from build123d import *

# Parameters (mm, degrees)
F0_R     = 31.75
F0_R_2   = 3.81
F1_DEPTH = 12.7
F4_DEPTH = 12.7
F5_COUNT = 20


with BuildPart() as f1:
    # F0 (on Front) → F1 (new body)
    with BuildSketch(Plane.XZ):
        Circle(F0_R)
        Circle(F0_R_2, mode=Mode.SUBTRACT)
    extrude(amount=F1_DEPTH)

    # F2 (on face) → F4 (join, through all)
    with BuildSketch(Plane.XZ.offset(12.7)):
        with BuildLine():
            Line((1.376606524, 33.9144617319), (0, 31.75))
            ThreePointArc((0, 31.75), (1.1215923583, 31.7301832737), (2.2417846354, 31.6707578319))
            Line((2.2417846354, 31.6707578319), (1.376606524, 33.9144617319))
        make_face()
    extrude(amount=-F4_DEPTH)

    # F5: F1 ×20 about axis
    f5_axis = Axis((0, -7.9411361367, 0), (0, -1, 0))


with BuildPart() as f1_1:
    add(f1.part)
    for i in range(1, F5_COUNT):
        add(f1.part.rotate(f5_axis, i * 360 / F5_COUNT))


solid = f1_1.part
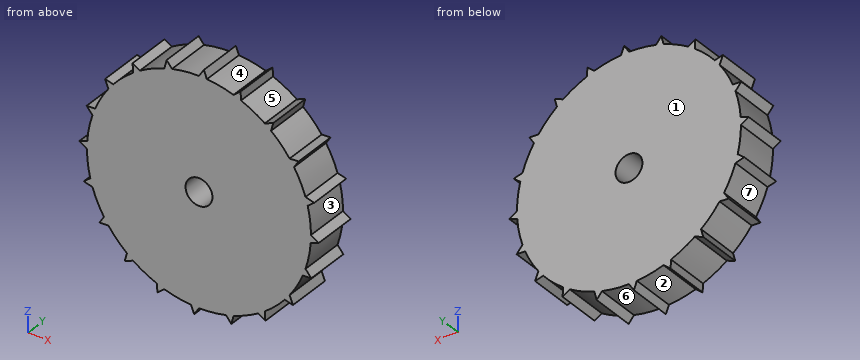
Build history of the part. All positions in model axes, mm. Face numbers are marked on the shaded views. A direction names the side the tool comes from. Coordinates: 2 decimals unless noted, no trailing zeros. Write each loop counter-clockwise with the first axis right and the second up, starting at its lowest first coordinate (ties: lowest second). Pieces come first, ordered by that corner, then holes.
(1) Pin check, flat tips, straight feed: pin 1 Ø1 at (y, z) = (-2, 4.5) entering from -X; pin 2 Ø1 at (x, y) = (18.5, -2.5) entering from +Z; pin 3 Ø1.5 at (y, z) = (-2.5, 27) entering from +X. Stop position of each tip, or through.
(2) Mould opens along Z. For the marked faces 1, 2, 3 and 4 say: pulls with the +Z half, pulls with the -Z half, needs draft (parallel to the pull), parting line crosses it, or undercut.
(3) Cut at A-A on z = -15.5. List the corners of the cut face in (x, y), and give its area (3 significant figures).
(4) Drill centre lines: line 1 (Z direction, x = 0, y = -9.75); line 2 (X direction, y = -3.25, z = -29.5); line 3 (X direction, y = -11, z = -13). Where is each one in solid material? Low to high.
(5) Cut at B-B on x = -5. List the corners of the cut face in (y, z).
(6) 3-axis set-ups, long thin cutter, end or side, ignore diameter. For the marked faces 5, 6 and 7: which of +Z, -Z, +X, -X, +Y, -Y reach the whole face in a straight line?
Working result:
1. pin 1: stops at x = -31.5
1. pin 2: stops at z = 26.15
1. pin 3: stops at x = 21.05
2. face 1: needs draft
2. face 2: pulls with the -Z half
2. face 3: undercut
2. face 4: pulls with the +Z half
3. outline: (-27.71, -12.7) - (27.71, -12.7) - (27.71, 0) - (-27.71, 0) - close
3. area: 704 mm2
4. line 1: z = -31.75 to -3.81, 3.81 to 31.75
4. line 2: x = -11.91 to 11.74
4. line 3: x = -28.97 to 28.97
5. outline: (-12.7, -31.35) - (0, -31.35) - (0, 31.35) - (-12.7, 31.35) - close
6. face 5: +Z, +Y, -Y
6. face 6: -Z, +Y, -Y
6. face 7: -X, +Y, -Y
